from build123d import *

# Parameters (mm, degrees)
SKETCH_R        = 65
PAD_DEPTH       = 3
SKETCH001_R     = 5
POCKET_DEPTH    = 1
SKETCH003_R     = 4
SKETCH003_R_2   = 1.5
PAD001_DEPTH    = 10
SKETCH005_R     = 50.047019
PAD002_DEPTH    = 2
SKETCH007_R     = 7.952006
POCKET001_DEPTH = 5


with BuildPart() as part:
    # Sketch → Pad (new body)
    with BuildSketch(Plane.XY):
        Circle(SKETCH_R)
    extrude(amount=PAD_DEPTH)

    # Sketch001 (on Face2 of Pad) → Pocket (cut)
    with BuildSketch(Plane(origin=(0, 0, 0), x_dir=(1, 0, 0), z_dir=(0, 0, -1))):
        with Locations((0, 45)):
            Circle(SKETCH001_R)
        with Locations((40.055428, -20.507625)):
            Circle(SKETCH001_R)
        with Locations((-40.055428, -20.507625)):
            Circle(SKETCH001_R)
    extrude(amount=-POCKET_DEPTH, mode=Mode.SUBTRACT)

    # Sketch003 (on Face3 of Pocket) → Pad001 (join)
    with BuildSketch(Plane.XY.offset(3)):
        with Locations((0, 40)):
            Circle(SKETCH003_R)
        with Locations((0, 40)):
            Circle(SKETCH003_R_2, mode=Mode.SUBTRACT)
        with Locations((-34.641016, -20)):
            Circle(SKETCH003_R)
        with Locations((-34.641016, -20)):
            Circle(SKETCH003_R_2, mode=Mode.SUBTRACT)
        with Locations((34.641016, -20)):
            Circle(SKETCH003_R)
        with Locations((34.641016, -20)):
            Circle(SKETCH003_R_2, mode=Mode.SUBTRACT)
    extrude(amount=PAD001_DEPTH)

    # Sketch005 (on Face15 of Pad001) → Pad002 (join)
    with BuildSketch(Plane.XY.offset(13)):
        Circle(SKETCH005_R)
    extrude(amount=PAD002_DEPTH)

    # Sketch007 (on Face3 of Pad002) → Pocket001 (cut)
    with BuildSketch(Plane.XY.offset(15)):
        Circle(SKETCH007_R)
    extrude(amount=-POCKET001_DEPTH, mode=Mode.SUBTRACT)


solid = part.part
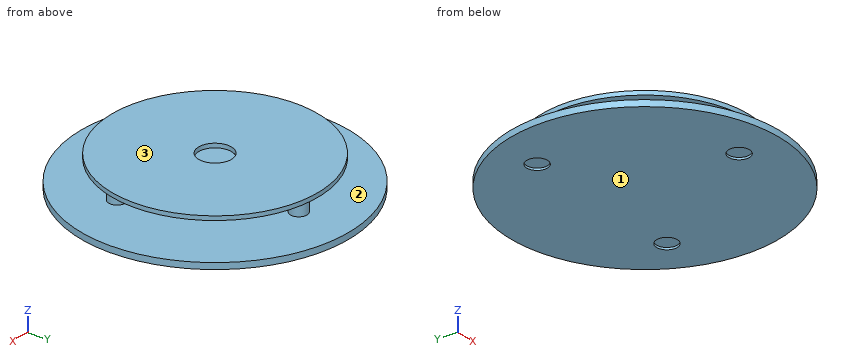
Check sheet for the modelled part. Datum: model origin and axes. Units: mm. Face numbers are marked on the shaded views. Round coordinates to 2 decimals unless told otherwise and drop trailing zeros. Loops run counter-clockwise (first coordinate to the right, second up) from the corner with the lowest first, then second, coordinate; pieces in that order, holes last. Notation, with made-up numbers: (33.25, 36) -> (42.25, 36) arc R18 ccw to (42.25, 66) -> close; hole circle Ø6 at (58, 39.5). An arc over 180 degrees is marked (long way). Put each result on its own line as item: value. Start each with the question number.
1. Draft check along Z on the marked faces 1, 2 and 3. Enter one of: +Z half, -Z half, draft (parallel to the pull), parting line (faces both ways), or undercut.
2. Section check D-D (x = -22). Enter the section's corners in (y, z).
3. Scan lines: probe 1 along Z at (x, y) = (15, 47); probe 2 along Y at (x, z) = (0, 0.5); probe 3 along Y at (x, z) = (0, 13.6). Record each from-to range of solid material in increasing order.
4. Section check B-B (z = 7.75). Enter the section's corners in (x, y), plus the area to 3 significant figures.
5. Gauge pin test, flat ends, axial feed: pin 1 (6 mm diameter, centred on x = 40.06, y = 20.51, fed in from -Z); pin 2 (8 mm diameter, centred on y = -50.5, z = 6, fed in from -X); pin 3 (6 mm diameter, centred on y = -45.5, z = 3.5, fed in from -X). Record the tip position at first contact, or that the pin passes through.
6. Section check A-A (x = 0). Enter the section's corners in (y, z), plus the area to 3 significant figures.
7. Section check C-C (y = 0). Enter the section's corners in (x, z).
Findings:
1. face 1: -Z half
1. face 2: undercut
1. face 3: +Z half
2. outline: (-61.16, 0) -> (61.16, 0) -> (61.16, 3) -> (-61.16, 3) -> close; (-44.95, 13) -> (44.95, 13) -> (44.95, 15) -> (-44.95, 15) -> close
3. probe 1: z = 0 to 3, 13 to 15
3. probe 2: y = -65 to -50, -40 to 65
3. probe 3: y = -50.05 to -7.95, 7.95 to 50.05
4. outline: circle Ø8 at (-34.64, -20); circle Ø8 at (0, 40); circle Ø8 at (34.64, -20); hole circle Ø3 at (-34.64, -20); hole circle Ø3 at (0, 40); hole circle Ø3 at (34.64, -20)
4. area: 130 mm^2
5. pin 1: stops at z = 1
5. pin 2: stops at x = -43.99
5. pin 3: stops at x = -49.14
6. outline: (-65, 0) -> (-50, 0) -> (-50, 1) -> (-40, 1) -> (-40, 0) -> (65, 0) -> (65, 3) -> (44, 3) -> (44, 13) -> (50.05, 13) -> (50.05, 15) -> (7.95, 15) -> (7.95, 13) -> (36, 13) -> (36, 3) -> (-65, 3) -> close; (-50.05, 13) -> (-7.95, 13) -> (-7.95, 15) -> (-50.05, 15) -> close; hole (38.5, 3) -> (41.5, 3) -> (41.5, 13) -> (38.5, 13) -> close
6. area: 598 mm^2
7. outline: (-65, 0) -> (65, 0) -> (65, 3) -> (-65, 3) -> close; (-50.05, 13) -> (-7.95, 13) -> (-7.95, 15) -> (-50.05, 15) -> close; (7.95, 13) -> (50.05, 13) -> (50.05, 15) -> (7.95, 15) -> close
